Here's how the part is built. I have some questions about the finished solid (model axes, mm). A direction names the side the tool comes from. Round coordinates to 2 decimals unless told otherwise and drop trailing zeros. Order: outer loops, then holes, each group sorted by start corner. A loop starts at its lowest first (then second) coordinate and runs counter-clockwise, first axis right, second up. Notation, with made-up numbers: M 82,53.25 L 134,53.25 A15 cw 134,61.25 Z; hole C 24.25,-16 d7. An arc over 180 degrees is marked long. Write item = value, one per line. Start each with the question number.
Item 1: I want a section at B-B, the plane z = -30. List the corners of the cut face in (x, y) for me, plus the area to 3 significant figures.
Item 2: I want a section at C-C, the plane x = -4. List the corners of the cut face in (y, z) for me.
Item 3: We'd pull the mould along Z, two halves only. Please class faces 3 (the face through (8, 10, 17.75)), 4 (the face through (-3, 20, 1)), 5 (the face through (0.23, 0.86, -39.1)), 6 (the face through (8, 10, -17.75)): pulls with the +Z half, pulls with the -Z half, needs draft (parallel to the pull), parting line crosses it, or undercut.
Item 4: I'm going to push flat-ended pins straight in: P1, Ø6, axis at y = 10.5, z = 1, coming from the +X side; P2, Ø5.5, axis at y = 10, z = 30, coming from the +X side. Where does each tip first touch, or does it pass through?
Item 5: Please list where these lines run through material, in increasing order: L1, parallel to Z at x = -7, y = 10; L2, parallel to Z at x = 5, y = 10; L3, parallel to Z at x = 15, y = 13.5.
Item 6: I want a section at A-A, the plane x = 7. List the corners of the cut face in (y, z) for me, plus the area to 3 significant figures.
Item 7: For faces 1 (the face through (-0.23, 19.1, 39.14)), 2 (the face through (-1, 10, 0)), which set-ups out of +Z, -Z, +X, -X, +Y, -Y let a thin tool reach every point of the face, with its end or its side?
Item 8: I want a section at D-D, the plane y = 5.25. List the corners of the cut face in (x, z) for me.
Autodesk Inventor part; units mm, degrees
ref_plane "YZ Plane" through (0, 0, 0) normal (1, 0, 0) x (0, 1, 0)
ref_plane "XZ Plane" through (0, 0, 0) normal (0, 1, 0) x (-1, 0, 0)
ref_plane "XY Plane" through (0, 0, 0) normal (0, 0, 1) x (1, 0, 0)
sketch "Sketch1" plane through (0, 0, 0) normal (0, 1, 0) x (-1, 0, 0)
  line L0 (-16.25, 40) -> (16.25, 40)
  line L1 (16.25, 40) -> (16.25, -40)
  line L2 (16.25, -40) -> (-16.25, -40)
  line L3 (-16.25, -40) -> (-16.25, 40)
  point P0 (0, 0)
  dimension "d0" = 80
  dimension "d1" = 32.5
  dimension "d2" = 40
  dimension "d3" = 16.25
extrude "Extrusion1" add sketch "Sketch1" along normal blind 20
sketch "Sketch2" plane through (16.25, 0, 40) normal (1, 0, 0) x (0, 0, -1)
  line L0 (0, 0) -> (80, 0)
  line L1 (80, 0) -> (80, 20)
  line L2 (0, 20) -> (80, 20)
  line L3 (0, 0) -> (0, 20)
  point P0 (40, 0)
  point P1 (10, 10)
  point P2 (70, 10)
  dimension "d8" = 10
  dimension "d9" = 10
  dimension "d10" = 10
  dimension "d11" = 10
hole "Hole1" at (16.25, 10, 30) at (16.25, 10, -30) direction (-1, 0, 0) diameter 6 end through all
sketch "Sketch3" plane through (0, 20, 0) normal (0, 1, 0) x (1, 0, 0)
  line L0 (16.25, -40) -> (16.25, 40)
  line L1 (16.25, 40) -> (-16.25, 40)
  line L2 (-16.25, 40) -> (-16.25, -40)
  line L3 (-16.25, -40) -> (16.25, -40)
  line L4 (16.25, -17.75) -> (-1, -17.75)
  line L5 (-1, -17.75) -> (-1, 17.75)
  line L6 (-1, 17.75) -> (16.25, 17.75)
  point P0 (0, 0)
  dimension "d19" = 17.25
  dimension "d20" = 35.5
  dimension "d21" = 17.75
extrude "Extrusion2" cut sketch "Sketch3" against normal through all contours L4 L5 L6 L0
fillet "Fillet1" radius 3 4 edges at (0, 20, 40) (0, 0, 40) (0, 20, -40) (0, 0, -40)
properties part number "3DP_ASA_Balcony_Mounting_Clamp_Back"
Filled in:
q1.outline = M -16.25,0 L 16.25,0 L 16.25,7 L -16.25,7 Z; M -16.25,13 L 16.25,13 L 16.25,20 L -16.25,20 Z
q1.area = 455 mm^2
q2.outline = M 0,-37 A3 ccw 3,-40 L 17,-40 A3 ccw 20,-37 L 20,37 A3 ccw 17,40 L 3,40 A3 ccw 0,37 Z; hole C 10,-30 d6; hole C 10,30 d6
q3.face_3 = undercut
q3.face_4 = needs draft
q3.face_5 = pulls with the -Z half
q3.face_6 = undercut
q4.P1 = -1
q4.P2 = through
q5.L1 = -40 to -33, -27 to 27, 33 to 40
q5.L2 = -40 to -33, -27 to -17.75, 17.75 to 27, 33 to 40
q5.L3 = -40 to -17.75, 17.75 to 40
q6.outline = M 0,-37 A3 ccw 3,-40 L 17,-40 A3 ccw 20,-37 L 20,-17.75 L 0,-17.75 Z; M 0,17.75 L 20,17.75 L 20,37 A3 ccw 17,40 L 3,40 A3 ccw 0,37 Z; hole C 10,-30 d6; hole C 10,30 d6
q6.area = 826 mm^2
q7.face_1 = +Z, +X, -X, +Y
q7.face_2 = +X, +Y, -Y
q8.outline = M -16.25,-40 L 16.25,-40 L 16.25,-17.75 L -1,-17.75 L -1,17.75 L 16.25,17.75 L 16.25,40 L -16.25,40 Z
